Autodesk Inventor part; units mm, degrees
ref_plane "YZ Plane" through (0, 0, 0) normal (1, 0, 0) x (0, 1, 0)
ref_plane "XZ Plane" through (0, 0, 0) normal (0, 1, 0) x (-1, 0, 0)
ref_plane "XY Plane" through (0, 0, 0) normal (0, 0, 1) x (1, 0, 0)
ref_plane "Arbeitsebene1" through (0, 0, 0) normal (0, 0, 1) x (1, 0, 0)
sketch "Skizze1" plane through (0, 0, 0) normal (0, 0, 1) x (1, 0, 0)
  circle A0 centre (34.3329, 7.5) radius 3.25 construction
  circle A1 centre (44.3329, 7.5) radius 3.25 construction
  circle A2 centre (34.3329, -7.5) radius 3.25 construction
  circle A3 centre (44.3329, -7.5) radius 3.25 construction
  line L0 (34.3329, 7.5) -> (44.3329, 7.5) construction
  line L1 (44.3329, 7.5) -> (44.3329, -7.5) construction
  line L2 (44.3329, -7.5) -> (34.3329, -7.5) construction
  line L3 (34.3329, -7.5) -> (34.3329, 7.5) construction
  line L4 (47.9329, 11.1) -> (30.7329, 11.1)
  line L5 (30.7329, 11.1) -> (30.7329, -11.1)
  line L6 (30.7329, -11.1) -> (47.9329, -11.1)
  line L7 (47.9329, -11.1) -> (47.9329, 11.1)
  circle A4 centre (34.3329, 7.5) radius 2.5
  circle A5 centre (44.3329, 7.5) radius 2.5
  circle A6 centre (34.3329, -7.5) radius 2.5
  circle A7 centre (44.3329, -7.5) radius 2.5
  point P0 (0, 0)
  dimension "d0" = 3.6
  dimension "d1" = 5
  dimension "d2" = 5
  dimension "d3" = 5
  dimension "d4" = 5
extrude "Extrusion1" add sketch "Skizze1" along normal blind 4
sketch "Skizze2" plane through (0, 0, 4) normal (0, 0, 1) x (1, 0, 0)
  line L0 (30.7329, 11.1) -> (30.7329, -11.1)
  line L1 (30.7329, -11.1) -> (47.9329, -11.1)
  line L2 (47.9329, -11.1) -> (47.9329, 11.1)
  line L3 (47.9329, 11.1) -> (30.7329, 11.1)
  circle A0 centre (34.3329, 7.5) radius 2.5
  circle A1 centre (44.3329, 7.5) radius 2.5
  circle A2 centre (34.3329, -7.5) radius 2.5
  circle A3 centre (44.3329, -7.5) radius 2.5
  point P0 (0, 0)
extrude "Extrusion2" add sketch "Skizze2" along normal blind 2 contours L3 L2 L1 L0 | A0 | A1 | A2 | A3
sketch "Skizze3" plane through (47.9329, -11.1, 0) normal (1, 0, 0) x (0, 0, -1)
  circle A0 centre (0, 11.1) radius 3.22
  circle A1 centre (0.7362, 11.1) radius 3.22
  point P0 (0, 11.1)
  dimension "d9" = 6.44
  dimension "d10" = 6.44
extrude "Extrusion3" cut sketch "Skizze3" against normal through all contours A0 A1 | A0 A1 picked at (-0.5511, 10.842) picked at (3.403, 11.6139)
fillet "Rundung1" radius 2 4 edges at (47.9329, -11.1, 3) (47.9329, 11.1, 3) (30.7329, 11.1, 3) (30.7329, -11.1, 3)
equation "\"d10\" = d9"
properties part number "20_Cube_Insert_Template_magnetic_clamp_v3"
The model under review builds one solid part; all positions refer to its coordinate system, in mm. A direction names the side the tool comes from. Round coordinates to 2 decimals unless told otherwise and drop trailing zeros. Loops run counter-clockwise (first coordinate to the right, second up) from the corner with the lowest first, then second, coordinate; pieces in that order, holes last. Notation, with made-up numbers: (66.25, 25) -> (85.25, 25) arc R15 ccw to (85.25, 51) -> close; hole circle Ø2 at (41.25, -18.75). An arc over 180 degrees is marked (long way). Answer as CSV lines item,"result".
1) Add section A-A on y = 7.5. Write out the cut boundary in (x, z).
Geometry results:
outline,"(30.73, 0) -> (31.83, 0) -> (31.83, 4) -> (36.83, 4) -> (36.83, 0) -> (41.83, 0) -> (41.83, 4) -> (46.83, 4) -> (46.83, 0) -> (47.93, 0) -> (47.93, 6) -> (30.73, 6) -> close"
2) To check wall thickness, follow line 1 along Y through (x, z) = (33.5, 0.6); line 2 along Y through (x, z) = (46, 0.3); line 3 along X through (y, z) = (7.75, 2.35). State the ranges of each line that lie inside material, in increasing order. Write a range as from..to.
Geometry results:
line 1,"y = -11.1..-9.86, -5.14..-2.93, 2.93..5.14, 9.86..11.1"
line 2,"y = -11.1..-9.36, -5.64..-3.05, 3.05..5.64, 9.36..11.1"
line 3,"x = 30.73..31.85, 36.82..41.85, 46.82..47.93"
3) For P1, Ø4.5, axis at x = 44.33, y = 7.5, coming from the -Z side, flat-tipped, find the tip position at first contact; note if it passes through.
Geometry results:
P1,"stops at z = 4"
4) Tool access review of faces 5 (the face through (44, 8, 4)), 6 (the face through (39, -7, 0)): name each direction out of +Z, -Z, +X, -X, +Y, -Y from which nothing blocks a thin tool from reaching the whole face with its end or side.
Geometry results:
face 5,"-Z"
face 6,"-Z, +X, -X, +Y, -Y"
5) Add section C-C on z = 3.1. Write out the cut boundary in (x, y).
Geometry results:
outline,"(30.73, -9.1) arc R2 ccw to (32.73, -11.1) -> (45.93, -11.1) arc R2 ccw to (47.93, -9.1) -> (47.93, 9.1) arc R2 ccw to (45.93, 11.1) -> (32.73, 11.1) arc R2 ccw to (30.73, 9.1) -> close; hole circle Ø5 at (34.33, -7.5); hole circle Ø5 at (34.33, 7.5); hole circle Ø5 at (44.33, -7.5); hole circle Ø5 at (44.33, 7.5)"
6) Add section D-D on x = 38.25. Write out the cut boundary in (y, z), plus the area to 3 significant figures.
Geometry results:
outline,"(-11.1, 0) -> (-3.13, 0) arc R3.22 cw to (3.13, 0) -> (11.1, 0) -> (11.1, 6) -> (-11.1, 6) -> close"
area,"122 mm²"
7) Add section B-B on z = 0.7. Write out the cut boundary in (x, y).
Geometry results:
outline,"(30.73, -9.1) arc R2 ccw to (32.73, -11.1) -> (45.93, -11.1) arc R2 ccw to (47.93, -9.1) -> (47.93, -2.88) -> (30.73, -2.88) -> close; (30.73, 2.88) -> (47.93, 2.88) -> (47.93, 9.1) arc R2 ccw to (45.93, 11.1) -> (32.73, 11.1) arc R2 ccw to (30.73, 9.1) -> close; hole circle Ø5 at (34.33, -7.5); hole circle Ø5 at (34.33, 7.5); hole circle Ø5 at (44.33, -7.5); hole circle Ø5 at (44.33, 7.5)"
8) Draft analysis for pull direction X (two halves, no side actions). For faces 1 (the face through (34, 8, 4)), 2 (the face through (30.733, 0, 3)), 3 (the face through (31.835, 7.39, 1.972)), 4 (the face through (39, 7, 0)), state which applies: pulls with the +X half, pulls with the -X half, needs draft (parallel to the pull), parting line crosses it, or undercut.
Geometry results:
face 1,"undercut"
face 2,"pulls with the -X half"
face 3,"undercut"
face 4,"needs draft"
